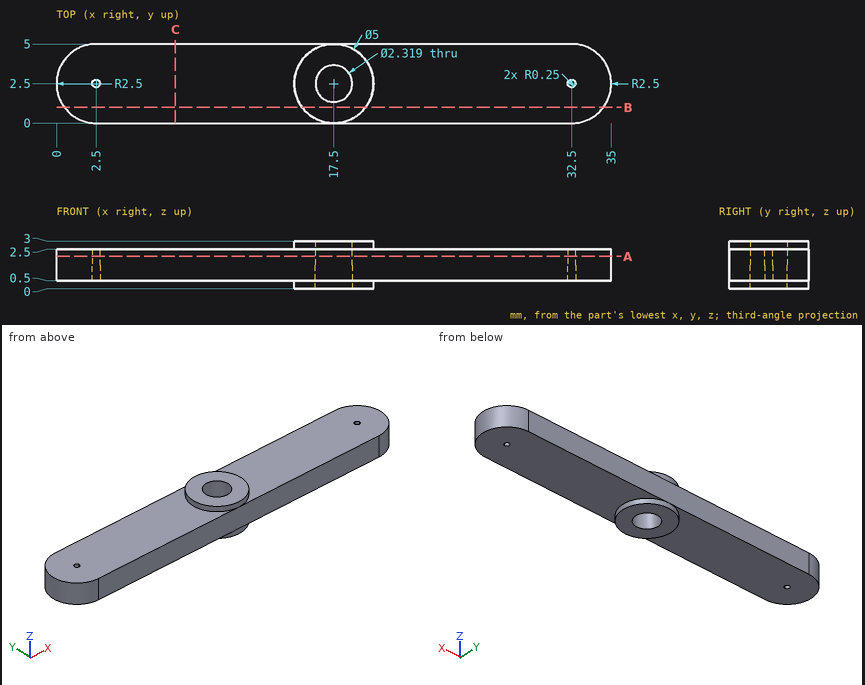
Source: three-view drawing plus pictorial views. Frame: mm from the lowest corner of the part. Round coordinates to 2 decimals unless told otherwise and drop trailing zeros. Loops run counter-clockwise (first coordinate to the right, second up) from the corner with the lowest first, then second, coordinate; pieces in that order, holes last. Notation, with made-up numbers: (71.5, 33) - (124.5, 33) arc R20 cw to (124.5, 52) - close; hole circle Ø4 at (-26, 35). An arc over 180 degrees is marked (long way). Write item = value, one per line. Start each with the question number.
Item 1: Section query A-A on z = 2.05. Output: boundary loops of the cut face in (x, y).
Item 2: First-contact query: pin 1 Ø2 at (x, y) = (17.5, 2.5) entering from +Z; pin 2 Ø1 at (x, y) = (11, 3) entering from +Z; pin 3 Ø2.5 at (x, y) = (23, 3) entering from -Z. Flat tips, straight axial feed; report the tip coordinate or a pass-through.
Item 3: Section query B-B on y = 1. Output: boundary loops of the cut face in (x, z), plus the area to 3 significant figures.
Item 4: Material intervals for line 1 (Y direction, x = 17.5, z = 0.8); line 2 (Z direction, x = 3, y = 0.4); line 3 (X direction, y = 1.8, z = 2.4), sorted ascending.
Item 5: Section query C-C on x = 7.5. Output: boundary loops of the cut face in (y, z), plus the area to 3 significant figures.
Results list:
q1.outline = (2.5, 0) - (32.5, 0) arc R2.5 ccw to (32.5, 5) - (2.5, 5) arc R2.5 ccw to start; hole circle Ø0.5 at (2.5, 2.5); hole circle Ø2.32 at (17.5, 2.5); hole circle Ø0.5 at (32.5, 2.5)
q2.pin_1 = through
q2.pin_2 = 2.5
q2.pin_3 = 0.5
q3.outline = (0.5, 0.5) - (15.5, 0.5) - (15.5, 0) - (19.5, 0) - (19.5, 0.5) - (34.5, 0.5) - (34.5, 2.5) - (19.5, 2.5) - (19.5, 3) - (15.5, 3) - (15.5, 2.5) - (0.5, 2.5) - close
q3.area = 72.0 mm²
q4.line_1 = 0 to 1.34, 3.66 to 5
q4.line_2 = 0.5 to 2.5
q4.line_3 = 0.1 to 16.58, 18.42 to 34.9
q5.outline = (0, 0.5) - (5, 0.5) - (5, 2.5) - (0, 2.5) - close
q5.area = 10.0 mm²
